from build123d import *

# Parameters (mm, degrees)
PAD_DEPTH        = 35
SKETCH001_R      = 3.15
POCKET_DEPTH     = 10
HOLE_D           = 3.2
HOLE_CSINK_D     = 6.1
HOLE_CSINK_ANGLE = 90


with BuildPart() as part:
    # Sketch → Pad (new body)
    with BuildSketch(Plane.XZ):
        Polygon((0, 0), (0, 67), (10, 67), (10, 8), (25, 8), (25, 0), align=None)
    extrude(amount=PAD_DEPTH)

    # Sketch001 → Pocket (cut)
    with BuildSketch(Plane.YZ):
        with Locations((-17.5, 49.5)):
            Circle(SKETCH001_R)
        with BuildLine():
            ThreePointArc((0, 49.5), (-17.5, 67), (-35, 49.5))
            Line((-35, 49.5), (-45, 49.5))
            Line((-45, 49.5), (-45, 74.5))
            Line((-45, 74.5), (10, 74.5))
            Line((10, 74.5), (10, 49.5))
            Line((10, 49.5), (0, 49.5))
        make_face()
    extrude(amount=POCKET_DEPTH, mode=Mode.SUBTRACT)

    # Hole (through all)
    with Locations(Plane(origin=(0, 0, 0), x_dir=(1, 0, 0), z_dir=(0, 0, -1))):
        with Locations((17.5, 8.75), (17.5, 26.25)):
            CounterSinkHole(HOLE_D / 2, HOLE_CSINK_D / 2, counter_sink_angle=HOLE_CSINK_ANGLE)


solid = part.part
Read the model definition and answer for the solid it produces. Units are mm, in the model's axes. A direction names the side the tool comes from. Coordinates: 2 decimals unless noted, no trailing zeros. Write each loop counter-clockwise with the first axis right and the second up, starting at its lowest first coordinate (ties: lowest second). Pieces come first, ordered by that corner, then holes. Notation, with made-up numbers: (-18.75, 24.5) -> (-8.75, 24.5) arc R20 cw to (-8.75, 52.5) -> close; hole circle Ø8 at (4, 27.5). An arc over 180 degrees is marked (long way). Return JSON: item names as keys, results as strings.
(1) For a pull along Z with two mould halves and no side action, classify faces 1 (the flat face through (13, -17, 0)), 2 (the cylindrical face through (4.93, -18.183, 46.425)), 3 (the flat face through (25, -17, 4)), 4 (the cylindrical face through (4.93, -17.115, 66.996)) as pulls with the +Z half, pulls with the -Z half, needs draft (parallel to the pull), parting line crosses it, or undercut.
Answers below:
{"face 1": "pulls with the -Z half", "face 2": "undercut", "face 3": "needs draft", "face 4": "pulls with the +Z half"}
(2) The part is cut by section B-B on x = 17.5. Give the vertices of the cut face in (y, z), then the cut area to 3 significant figures.
Answers below:
{"outline": "(-35, 0) -> (-29.3, 0) -> (-27.85, 1.45) -> (-27.85, 8) -> (-35, 8) -> close; (-24.65, 1.45) -> (-23.2, 0) -> (-11.8, 0) -> (-10.35, 1.45) -> (-10.35, 8) -> (-24.65, 8) -> close; (-7.15, 1.45) -> (-5.7, 0) -> (0, 0) -> (0, 8) -> (-7.15, 8) -> close", "area": "225 mm^2"}
(3) The part is cut by section C-C on z = 51. Give the vertices of the cut face in (x, y), then the cut area to 3 significant figures.
Answers below:
{"outline": "(0, -34.94) -> (10, -34.94) -> (10, -20.27) -> (0, -20.27) -> close; (0, -14.73) -> (10, -14.73) -> (10, -0.06) -> (0, -0.06) -> close", "area": "293 mm^2"}
(4) The part is cut by section D-D on z = 17.5. Give the vertices of the cut face in (x, y), then the cut area to 3 significant figures.
Answers below:
{"outline": "(0, -35) -> (10, -35) -> (10, 0) -> (0, 0) -> close", "area": "350 mm^2"}
(5) The part is cut by section A-A on y = -17.5. Give the vertices of the cut face in (x, z), then the cut area to 3 significant figures.
Answers below:
{"outline": "(0, 0) -> (25, 0) -> (25, 8) -> (10, 8) -> (10, 46.35) -> (0, 46.35) -> close; (0, 52.65) -> (10, 52.65) -> (10, 67) -> (0, 67) -> close", "area": "727 mm^2"}
(6) Each of these flat-tipped pins is pushed along its axis until it touches: P1, Ø10, axis at x = 6.5, y = -28.5, coming from the +Z side; P2, Ø5, axis at x = 17.5, y = -26.25, coming from the +Z side. Where does it stop, or does it pass through?
Answers below:
{"P1": "z = 65.94", "P2": "z = 8"}
(7) Consider line 1 along Y through (x, z) = (17.5, 6.75); line 2 along X through (y, z) = (-8.75, 6); line 3 along Z through (x, y) = (5.25, -17.5). Determine where each line is inside the solid, lowest interval first. Write a range as from..to.
Answers below:
{"line 1": "-35..-27.85, -24.65..-10.35, -7.15..0", "line 2": "0..15.9, 19.1..25", "line 3": "0..46.35, 52.65..67"}
(8) Which of the six approach directions +Z, -Z, +X, -X, +Y, -Y give full straight-line access (tool end or side, diameter ignored) to faces 5 (the flat face through (10, -17, 38)), 6 (the flat face through (7, 0, 25))?
Answers below:
{"face 5": "+Z, +X, +Y, -Y", "face 6": "+Z, -Z, +X, -X, +Y"}
